```python
from build123d import *

# Parameters (mm, degrees)
SKETCH1_W           = 177.8
SKETCH1_H           = 127
BOSS_EXTRUDE1_DEPTH = 86.36
SKETCH2_R           = 29.337
CUT_EXTRUDE1_DEPTH  = 19.05
SHELL1_T            = -6.35
SKETCH4_R           = 12.7
CUT_EXTRUDE2_DEPTH  = 6.35


with BuildPart() as part:
    # Sketch1 → Boss-Extrude1 (new body)
    with BuildSketch(Plane(origin=(0, 0, 0), x_dir=(1, 0, 0), z_dir=(0, 1, 0))):
        Rectangle(SKETCH1_W, SKETCH1_H)
    extrude(amount=BOSS_EXTRUDE1_DEPTH)

    # Sketch2 → Cut-Extrude1 (cut)
    with BuildSketch(Plane(origin=(0, 86.36, 0), x_dir=(1, 0, 0), z_dir=(0, 1, 0))):
        with Locations(Location((0, 0, 0), (0, 0, 270))):
            Circle(SKETCH2_R)
    extrude(amount=-CUT_EXTRUDE1_DEPTH, mode=Mode.SUBTRACT)

    # Shell1
    shell1_openings = [part.faces().sort_by_distance(p)[0] for p in [
        (0, 0, 0),
    ]]
    offset(amount=SHELL1_T, openings=shell1_openings, kind=Kind.INTERSECTION)

    # Sketch4 → Cut-Extrude2 (cut)
    with BuildSketch(Plane.XZ.offset(-60.96)):
        with Locations(Location((0, 0, 0), (0, 0, 270))):
            Circle(SKETCH4_R)
    extrude(amount=-CUT_EXTRUDE2_DEPTH, mode=Mode.SUBTRACT)


solid = part.part
```
The listing builds one solid part. Answer for the finished solid, in the listing's coordinates (mm). A direction names the side the tool comes from. Round coordinates to 2 decimals unless told otherwise and drop trailing zeros. Write each loop counter-clockwise with the first axis right and the second up, starting at its lowest first coordinate (ties: lowest second). Pieces come first, ordered by that corner, then holes. Notation, with made-up numbers: (67.5, 76) -> (125.5, 76) arc R28 ccw to (125.5, 106) -> close; hole circle Ø10 at (8, -24). An arc over 180 degrees is marked (long way). Answer as a JSON object with one key per item and string values. Group by question number.
Q1. Determine the mould class of faces 1 (the face through (88.9, 43, 1)), 2 (the face through (-7.7, 64.1, 10.1)), 3 (the face through (-1, 43, -63.5)) for opening direction X: pulls with the +X half, pulls with the -X half, needs draft (parallel to the pull), parting line crosses it, or undercut.
Q2. Straight lines are drawn through the part: line 1 along X through (y, z) = (79.75, 0); line 2 along X through (y, z) = (62.5, 0); line 3 along Z through (x, y) = (-60.5, 72). For each, find the intervals that lie inside material, in ascending order.
Q3. Section C-C (x = 0) is taken. Write down the section's boundary in (y, z), plus the area to 3 significant figures.
Q4. Section B-B (z = 0) is taken. Write down the section's boundary in (x, y).
Q5. Section A-A (y = 77) is taken. Write down the section's boundary in (x, z), plus the area to 3 significant figures.
Q6. Each of these flat-tipped pins is pushed along its axis until it touches: pin 1 Ø12 at (x, z) = (-57.5, -16) entering from -Y; pin 2 Ø3 at (x, z) = (10, -9) entering from -Y. Where does it stop, or does it pass through?
Q7. Section D-D (x = -41.5) is taken. Write down the section's boundary in (y, z).
Q8. Which of the six approach directions +Z, -Z, +X, -X, +Y, -Y give full straight-line access (tool end or side, diameter ignored) to faces 4 (the face through (-6, 67.31, 13)), 5 (the face through (82.55, 39, 1)), 6 (the face through (-88.9, 43, 1))?
Check values:
{
 "1": {"face 1": "pulls with the +X half", "face 2": "undercut", "face 3": "needs draft"},
 "2": {"line 1": "-88.9 to -82.55, -35.69 to -29.34, 29.34 to 35.69, 82.55 to 88.9", "line 2": "-88.9 to -82.55, -35.69 to -12.7, 12.7 to 35.69, 82.55 to 88.9", "line 3": "-63.5 to -57.15, 57.15 to 63.5"},
 "3": {"outline": "(0, -63.5) -> (86.36, -63.5) -> (86.36, -29.34) -> (67.31, -29.34) -> (67.31, -12.7) -> (60.96, -12.7) -> (60.96, -35.69) -> (80.01, -35.69) -> (80.01, -57.15) -> (0, -57.15) -> close; (0, 57.15) -> (80.01, 57.15) -> (80.01, 35.69) -> (60.96, 35.69) -> (60.96, 12.7) -> (67.31, 12.7) -> (67.31, 29.34) -> (86.36, 29.34) -> (86.36, 63.5) -> (0, 63.5) -> close", "area": "1,900 mm^2"},
 "4": {"outline": "(-88.9, 0) -> (-82.55, 0) -> (-82.55, 80.01) -> (-35.69, 80.01) -> (-35.69, 60.96) -> (-12.7, 60.96) -> (-12.7, 67.31) -> (-29.34, 67.31) -> (-29.34, 86.36) -> (-88.9, 86.36) -> close; (12.7, 60.96) -> (35.69, 60.96) -> (35.69, 80.01) -> (82.55, 80.01) -> (82.55, 0) -> (88.9, 0) -> (88.9, 86.36) -> (29.34, 86.36) -> (29.34, 67.31) -> (12.7, 67.31) -> close"},
 "5": {"outline": "(-88.9, -63.5) -> (88.9, -63.5) -> (88.9, 63.5) -> (-88.9, 63.5) -> close; circle Ø71.37 at (0, 0); hole (-82.55, -57.15) -> (82.55, -57.15) -> (82.55, 57.15) -> (-82.55, 57.15) -> close; hole circle Ø58.67 at (0, 0)", "area": "5,010 mm^2"},
 "6": {"pin 1": "y = 80.01", "pin 2": "y = 60.96"},
 "7": {"outline": "(0, -63.5) -> (86.36, -63.5) -> (86.36, 63.5) -> (0, 63.5) -> (0, 57.15) -> (80.01, 57.15) -> (80.01, -57.15) -> (0, -57.15) -> close"},
 "8": {"face 4": "+Y", "face 5": "-Y", "face 6": "+Z, -Z, -X, +Y, -Y"}
}
